Check sheet for the modelled part. Datum: model origin and axes. Units: mm. A direction names the side the tool comes from. Coordinates: 2 decimals unless noted, no trailing zeros. Order: outer loops, then holes, each group sorted by start corner. A loop starts at its lowest first (then second) coordinate and runs counter-clockwise, first axis right, second up.
1. Thickness scan on line 1 (Y direction, x = 5, z = 0) (3 decimals); line 2 (Z direction, x = 6.25, y = 3); line 3 (X direction, y = 15.5, z = 18.5) (3 decimals). Record the ranges inside material, lowest first.
2. Gauge pin test, flat ends, axial feed: pin 1 Ø4 at (x, z) = (8, -9) entering from -Y; pin 2 Ø1.5 at (x, z) = (8, -12) entering from +Y; pin 3 Ø5 at (x, y) = (4, -12) entering from +Z. Record the tip position at first contact, or that the pin passes through.
3. Cross-section at D-D (z = -16.5). Enter the section's corners in (x, y) (3 decimals).
4. Cross-section at C-C (x = 8.25). Enter the section's corners in (y, z) (3 decimals), then the cut area to 3 significant figures.
5. Cross-section at A-A (y = 0). Enter the section's corners in (x, z) (3 decimals).
6. Draft check along Z on faces 1 (the cylindrical face through (7.826, -5.796, -7.559)), 2 (the flat face through (15.875, -10, 0)), 3 (the cylindrical face through (9.436, 6.676, -21.199)). Enter one of: released by +Z, released by -Z, zero draft, split by the parting line, or undercut.
7. Set-up check for faces 4 (the flat face through (0, 0, -11)), 5 (the flat face through (3.175, -22.5, 0.1)): record each of +Z, -Z, +X, -X, +Y, -Y from which the full face is reachable in a straight line by a thin tool's end or side.
```python
from build123d import *

# Parameters (mm, degrees)
SKETCH1_R           = 25.4
BOSS_EXTRUDE1_DEPTH = 3.175
SKETCH2_R           = 22.225
BOSS_EXTRUDE2_DEPTH = 12.7
SKETCH3_R           = 9.525
CUT_EXTRUDE1_DEPTH  = 16.875


with BuildPart() as part:
    # Sketch1 → Boss-Extrude1 (new body)
    with BuildSketch(Plane(origin=(0, 0, 0), x_dir=(0, 0, -1), z_dir=(1, 0, 0))):
        Circle(SKETCH1_R)
    extrude(amount=BOSS_EXTRUDE1_DEPTH)

    # Sketch2 → Boss-Extrude2 (add)
    with BuildSketch(Plane(origin=(3.175, 0, 0), x_dir=(0, 0, -1), z_dir=(1, 0, 0))):
        Circle(SKETCH2_R)
    extrude(amount=BOSS_EXTRUDE2_DEPTH)

    # Sketch3 → Cut-Extrude1 (cut, through all)
    with BuildSketch(Plane.ZY):
        Circle(SKETCH3_R)
    extrude(amount=-CUT_EXTRUDE1_DEPTH, mode=Mode.SUBTRACT)


solid = part.part
```
Data:
1. line 1: y = -22.225 to -9.525, 9.525 to 22.225
1. line 2: z = -22.02 to -9.04, 9.04 to 22.02
1. line 3: x = 0 to 3.175
2. pin 1: stops at y = -21.09
2. pin 2: stops at y = 19.17
2. pin 3: stops at z = 23.5
3. outline: (0, -19.311) - (3.175, -19.311) - (3.175, -14.89) - (15.875, -14.89) - (15.875, 14.89) - (3.175, 14.89) - (3.175, 19.311) - (0, 19.311) - close
4. outline: circle Ø44.45 at (0, 0); hole circle Ø19.05 at (0, 0)
4. area: 1,270 mm2
5. outline: (0, -25.4) - (3.175, -25.4) - (3.175, -22.225) - (15.875, -22.225) - (15.875, -9.525) - (0, -9.525) - close; (0, 9.525) - (15.875, 9.525) - (15.875, 22.225) - (3.175, 22.225) - (3.175, 25.4) - (0, 25.4) - close
6. face 1: undercut
6. face 2: zero draft
6. face 3: split by the parting line
7. face 4: +Z, -Z, -X, +Y, -Y
7. face 5: +X
